Design review of the part built by this model. Coordinates are the model's own, in mm. Coordinates: 2 decimals unless noted, no trailing zeros. Write each loop counter-clockwise with the first axis right and the second up, starting at its lowest first coordinate (ties: lowest second). Pieces come first, ordered by that corner, then holes.
Q1. Take a section at A-A, the plane y = 0. Write out the cut boundary in (x, z).
Q2. For pin 1 Ø2 at (x, z) = (3, -19) entering from -Y, flat-tipped, find the tip position at first contact; note if it passes through.
Q3. Take a section at B-B, the plane z = 208. Write out the cut boundary in (x, y).
Q4. For L1, parallel to X at y = 0, z = 219; L2, parallel to Y at x = 0, z = -109; L3, parallel to Y at x = -0.25, z = 90, list the stretches that pass through material, from the lowest coordinate up.
Autodesk Inventor part; units mm, degrees
ref_plane "YZ Plane" through (0, 0, 0) normal (1, 0, 0) x (0, 1, 0)
ref_plane "XZ Plane" through (0, 0, 0) normal (0, 1, 0) x (-1, 0, 0)
ref_plane "XY Plane" through (0, 0, 0) normal (0, 0, 1) x (1, 0, 0)
sketch "Sketch1" plane through (0, 0, 0) normal (0, 0, 1) x (1, 0, 0)
  line L0 (-6.35, -3.6662) -> (-6.35, 3.6662)
  line L1 (-6.35, 3.6662) -> (0, 7.3323)
  line L2 (0, 7.3323) -> (6.35, 3.6662)
  line L3 (6.35, 3.6662) -> (6.35, -3.6662)
  line L4 (6.35, -3.6662) -> (0, -7.3323)
  line L5 (0, -7.3323) -> (-6.35, -3.6662)
  point P0 (0, 0)
  point P1 (0, 0)
  dimension "Size" = 12.7
extrude "Extrusion1" add sketch "Sketch1" along normal mid plane 533.4
sketch "Sketch3" plane through (0, 0, 266.7) normal (0, 0, 1) x (1, 0, 0)
  line L0 (-6.35, 3.6662) -> (0, 7.3323) construction
  line L1 (0, 7.3323) -> (6.35, 3.6662) construction
  line L2 (6.35, 3.6662) -> (6.35, -3.6662) construction
  line L3 (6.35, -3.6662) -> (0, -7.3323) construction
  line L4 (0, -7.3323) -> (-6.35, -3.6662) construction
  line L5 (-6.35, -3.6662) -> (-6.35, 3.6662) construction
  point P0 (0, 0)
hole "Hole1" at (0, 0, 266.7) direction (0, 0, -1) diameter 5.1054 end through all
sketch "Sketch4" plane through (0, 0, 266.7) normal (0, 0, 1) x (1, 0, 0)
  circle A0 centre (0, 0) radius 2.5527 construction
  line L0 (-6.35, 3.6662) -> (0, 7.3323) construction
  line L1 (0, 7.3323) -> (6.35, 3.6662) construction
  line L2 (6.35, 3.6662) -> (6.35, -3.6662) construction
  line L3 (6.35, -3.6662) -> (0, -7.3323) construction
  line L4 (0, -7.3323) -> (-6.35, -3.6662) construction
  line L5 (-6.35, -3.6662) -> (-6.35, 3.6662) construction
  circle A1 centre (0, 0) radius 6.8771
  circle A2 centre (0, 0) radius 8.89
  dimension "thunder" = 13.7541
  dimension "d16" = 17.78
extrude "Extrusion3" cut sketch "Sketch4" against normal through all
equation "\"bearing\" = 25.4"
properties part number "GI - 002" material "Aluminum 6061"
Responses:
1. outline: (-6.35, -266.7) - (-2.55, -266.7) - (-2.55, 266.7) - (-6.35, 266.7) - close; (2.55, -266.7) - (6.35, -266.7) - (6.35, 266.7) - (2.55, 266.7) - close
2. pin 1: stops at y = -6.18
3. outline: (-6.35, -2.64) arc R6.88 ccw to (-5.46, -4.18) - (-0.89, -6.82) arc R6.88 ccw to (0.89, -6.82) - (5.46, -4.18) arc R6.88 ccw to (6.35, -2.64) - (6.35, 2.64) arc R6.88 ccw to (5.46, 4.18) - (0.89, 6.82) arc R6.88 ccw to (-0.89, 6.82) - (-5.46, 4.18) arc R6.88 ccw to (-6.35, 2.64) - close; hole circle Ø5.11 at (0, 0)
4. L1: x = -6.35 to -2.55, 2.55 to 6.35
4. L2: y = -6.88 to -2.55, 2.55 to 6.88
4. L3: y = -6.87 to -2.54, 2.54 to 6.87
